Print and shaded views of the part. All mm, measured from the part's lowest x, y and z. A direction names the side the tool comes from. Coordinates: 2 decimals unless noted, no trailing zeros. Order: outer loops, then holes, each group sorted by start corner. A loop starts at its lowest first (then second) coordinate and runs counter-clockwise, first axis right, second up. Notation, with made-up numbers: M 66,87.25 L 109,87.25 A24 ccw 109,126.25 Z; hole C 53,49 d4. An arc over 180 degrees is marked long. Use a Markdown table: item, result. Add a question column.
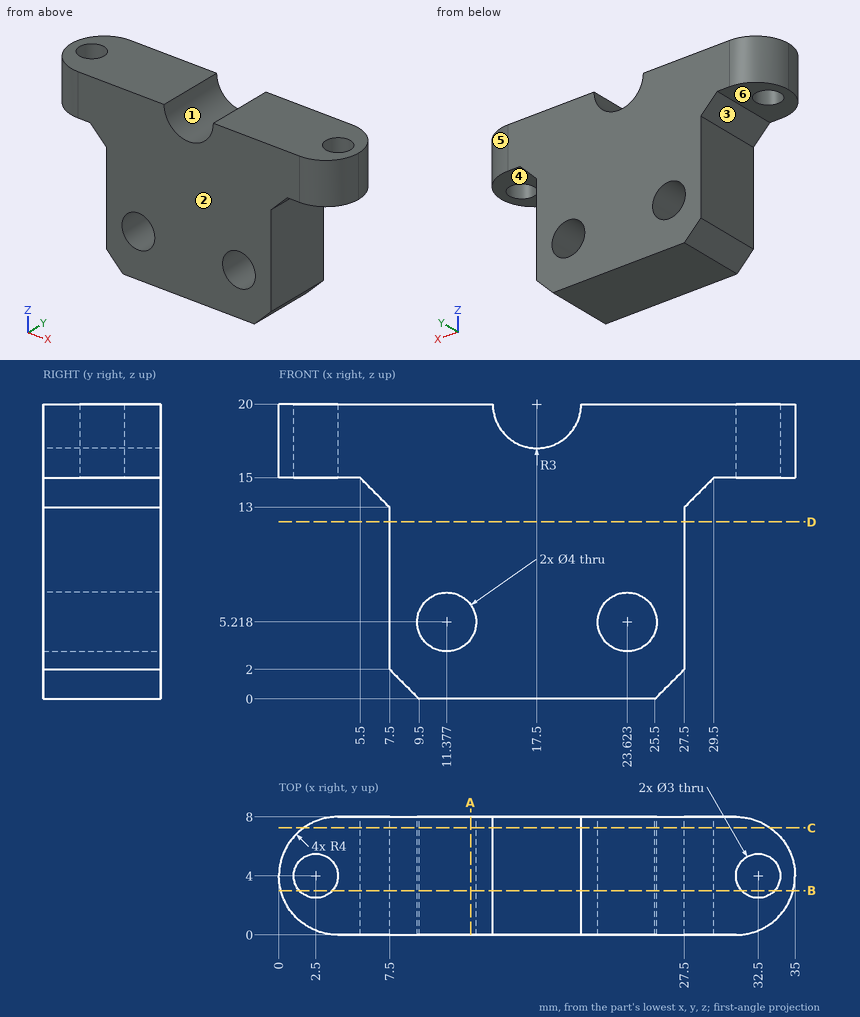
(1) Which spindle directions (+Z, -Z, +X, -X, +Y, -Y) get a long thin tool onto all of the face, cutting with end or side? Do the marked faces 4, 5 and 6. Say none if no direction does.
(2) Drop flat-ended pins along their axis: P1, Ø4, axis at y = 1.5, z = 6.5, coming from the +X side; P2, Ø1.6, axis at x = 1.5, y = 4, coming from the -Z side; P3, Ø1.5, axis at y = 5, z = 7.5, coming from the -X side; P4, Ø2.5, axis at x = 2.5, y = 4, coming from the -Z side. Give the stop position or say it passes through.
(3) Slice it at B-B on y = 3. Give the cut face in (x, z).
(4) Slice it at A-A on x = 13. Give the cut face in (y, z), and give its area (3 significant figures).
(5) Drill centre lines: line 1 along X through (y, z) = (6, 5.5); line 2 along X through (y, z) = (3.5, 17.25) (1 decimal); line 3 along X through (y, z) = (3.25, 2). Where is each one in solid material? Low to high. Write a range as from..to.
(6) Mould opens along X. For the marked faces 1, 2 and 3 say: released by +X, released by -X, zero draft, split by the parting line, or undercut.
(7) Slice it at D-D on z = 12. Give the cut face in (x, y), and give its area (3 significant figures).
(8) Slice it at C-C on y = 7.25. Give the cut face in (x, z).
Solutions:
| question | item | result |
|---|---|---|
| 1 | face 4 | -Z, +X, +Y, -Y |
| 1 | face 5 | +Z, -Z, +X, +Y |
| 1 | face 6 | -Z, -X, +Y, -Y |
| 2 | P1 | x = 27.5 |
| 2 | P2 | z = 15 |
| 2 | P3 | x = 7.5 |
| 2 | P4 | through |
| 3 | outline | M 0.13,15 L 1.38,15 L 1.38,20 L 0.13,20 Z; M 3.62,15 L 5.5,15 L 7.5,13 L 7.5,2 L 9.5,0 L 25.5,0 L 27.5,2 L 27.5,13 L 29.5,15 L 31.38,15 L 31.38,20 L 20.5,20 A3 cw 14.5,20 L 3.62,20 Z; M 33.62,15 L 34.87,15 L 34.87,20 L 33.62,20 Z; hole C 11.38,5.22 d4; hole C 23.62,5.22 d4 |
| 4 | outline | M 0,0 L 8,0 L 8,4.05 L 0,4.05 Z; M 0,6.39 L 8,6.39 L 8,20 L 0,20 Z |
| 4 | area | 141 mm² |
| 5 | line 1 | 7.5..9.4, 13.36..21.64, 25.6..27.5 |
| 5 | line 2 | 0..1.1, 3.9..16.3, 18.7..31.1, 33.9..35 |
| 5 | line 3 | 7.5..27.5 |
| 6 | face 1 | undercut |
| 6 | face 2 | zero draft |
| 6 | face 3 | released by -X |
| 7 | outline | M 7.5,0 L 27.5,0 L 27.5,8 L 7.5,8 Z |
| 7 | area | 160 mm² |
| 8 | outline | M 1.67,15 L 5.5,15 L 7.5,13 L 7.5,2 L 9.5,0 L 25.5,0 L 27.5,2 L 27.5,13 L 29.5,15 L 33.33,15 L 33.33,20 L 20.5,20 A3 cw 14.5,20 L 1.67,20 Z; hole C 11.38,5.22 d4; hole C 23.62,5.22 d4 |
